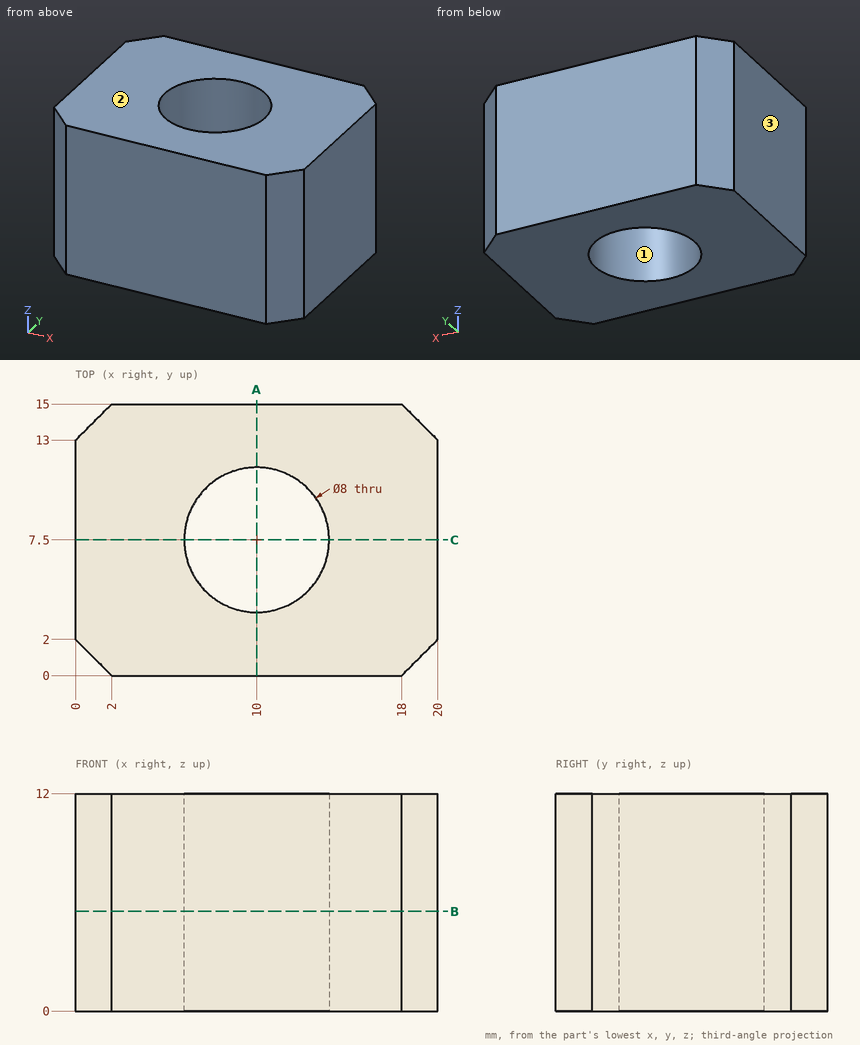
Geometry: see drawing. Coordinates: mm, zero at the bounding-box minimum. Round coordinates to 2 decimals unless told otherwise and drop trailing zeros. Order: outer loops, then holes, each group sorted by start corner. A loop starts at its lowest first (then second) coordinate and runs counter-clockwise, first axis right, second up. Notation, with made-up numbers: (71, 65.5) -> (111, 65.5) arc R20 ccw to (111, 104.5) -> close; hole circle Ø11 at (-13, 38.5). An arc over 180 degrees is marked (long way). Use CSV: the item, a comma, the result in double quotes.
(1) Pull-direction query (X, two-part tool) for the marked faces 1, 2 and 3; classes: +X half, -X half, draft (parallel to the pull), parting line (faces both ways), or undercut.
Report:
face 1,"undercut"
face 2,"draft"
face 3,"-X half"
(2) Section B-B on z = 5.5. Return the cut outline in (x, y).
Report:
outline,"(0, 2) -> (2, 0) -> (18, 0) -> (20, 2) -> (20, 13) -> (18, 15) -> (2, 15) -> (0, 13) -> close; hole circle Ø8 at (10, 7.5)"
(3) Ray query, L1, parallel to Y at x = 10, z = 3; L2, parallel to X at y = 4.75, z = 11.5; L3, parallel to Y at x = 11.25, z = 6.5. Return the intervals inside material, ascending.
Report:
L1,"0 to 3.5, 11.5 to 15"
L2,"0 to 7.1, 12.9 to 20"
L3,"0 to 3.7, 11.3 to 15"
(4) Section A-A on x = 10. Return the cut outline in (y, z).
Report:
outline,"(0, 0) -> (3.5, 0) -> (3.5, 12) -> (0, 12) -> close; (11.5, 0) -> (15, 0) -> (15, 12) -> (11.5, 12) -> close"
(5) Section C-C on y = 7.5. Return the cut outline in (x, z), and give its area (3 significant figures).
Report:
outline,"(0, 0) -> (6, 0) -> (6, 12) -> (0, 12) -> close; (14, 0) -> (20, 0) -> (20, 12) -> (14, 12) -> close"
area,"144 mm^2"
